Answer from the drawing. Dimensions are ordinates in mm from the lowest x, y and z of the part. A direction names the side the tool comes from. Coordinates: 2 decimals unless noted, no trailing zeros. Order: outer loops, then holes, each group sorted by start corner. A loop starts at its lowest first (then second) coordinate and runs counter-clockwise, first axis right, second up. Notation, with made-up numbers: (8.25, 60) -> (30.25, 60) arc R22 ccw to (30.25, 88) -> close; hole circle Ø3 at (51, -15). An arc over 180 degrees is marked (long way). Use CSV: the item, a comma, the result in double quotes.
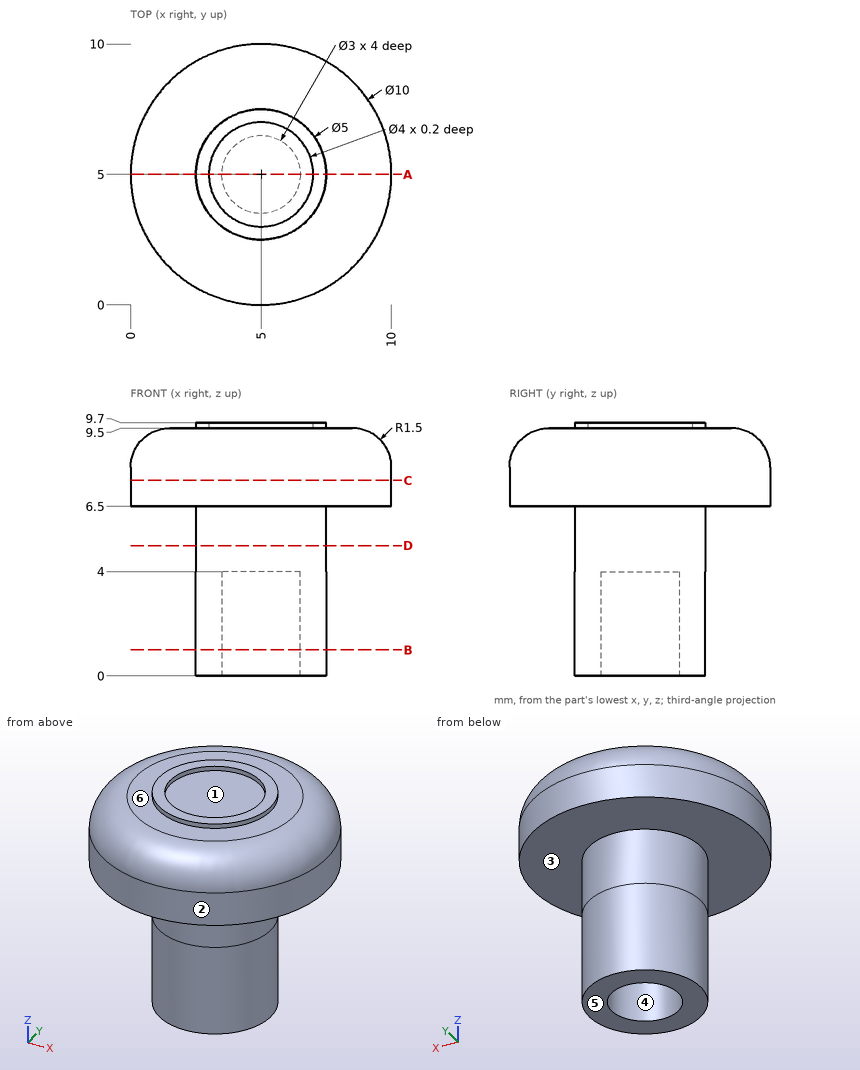
Item 1: A tool of negligible diameter and unlimited length cuts with its end or side. For the marked faces 4, 5 and 6, from which of +Z, -Z, +X, -X, +Y, -Y can it reach the whole face along a straight path? Write none if from no direction.
Return value:
face 4,"-Z"
face 5,"-Z, +X, -X, +Y, -Y"
face 6,"+Z"
Item 2: Find section C-C, the plane z = 7.5. Give the vertices of the cut face in (x, y).
Return value:
outline,"circle Ø10 at (5, 5)"
Item 3: The mould has two halves that part along X. Classify the marked faces 1, 2 and 3: +X half, -X half, draft (parallel to the pull), parting line (faces both ways), or undercut.
Return value:
face 1,"undercut"
face 2,"parting line"
face 3,"draft"
Item 4: Find section A-A, the plane y = 5. Give the vertices of the cut face in (x, z), then the cut area to 3 significant figures.
Return value:
outline,"(0, 6.5) -> (2.5, 6.5) -> (2.5, 0) -> (3.5, 0) -> (3.5, 4) -> (6.5, 4) -> (6.5, 0) -> (7.5, 0) -> (7.5, 6.5) -> (10, 6.5) -> (10, 8) arc R1.5 ccw to (8.5, 9.5) -> (7.5, 9.5) -> (7.5, 9.7) -> (7, 9.7) -> (7, 9.5) -> (3, 9.5) -> (3, 9.7) -> (2.5, 9.7) -> (2.5, 9.5) -> (1.5, 9.5) arc R1.5 ccw to (0, 8) -> close"
area,"49.7 mm^2"
Item 5: Find section D-D, the plane z = 5. Give the vertices of the cut face in (x, y).
Return value:
outline,"circle Ø5 at (5, 5)"
Item 6: Find section B-B, the plane z = 1. Give the vertices of the cut face in (x, y).
Return value:
outline,"circle Ø5 at (5, 5); hole circle Ø3 at (5, 5)"
Item 7: Straight lines are drawn through the part: line 1 along X through (y, z) = (5, 1.8); line 2 along Y through (x, z) = (5, 9.65). For each, find the intervals that lie inside material, in ascending order.
Return value:
line 1,"x = 2.5 to 3.5, 6.5 to 7.5"
line 2,"y = 2.5 to 3, 7 to 7.5"
Item 8: Each of these flat-tipped pins is pushed along its axis until it touches: P1, Ø1, axis at x = 1, y = 2, coming from the +Z side; P2, Ø5, axis at x = 7.5, z = 1, coming from the +Y side. Where does it stop, or does it pass through?
Return value:
P1,"stops at z = 9.12"
P2,"stops at y = 7.5"
